from build123d import *

# Parameters (mm, degrees)
SKETCH1_W           = 250
SKETCH1_H           = 150
SKETCH1_R           = 6
BOSS_EXTRUDE1_DEPTH = 9.525
SKETCH2_W           = 9.525
SKETCH2_H           = 150
BOSS_EXTRUDE2_DEPTH = 200
SKETCH3_W           = 9.525
SKETCH3_H           = 150
BOSS_EXTRUDE3_DEPTH = 150


with BuildPart() as part:
    # Sketch1 → Boss-Extrude1 (new body)
    with BuildSketch(Plane.XY):
        with Locations((125, -75)):
            Rectangle(SKETCH1_W, SKETCH1_H)
        with Locations(Location((53.75, -40.75, 0), (0, 0, 180))):
            Circle(SKETCH1_R, mode=Mode.SUBTRACT)
        with Locations(Location((196.25, -40.75, 0), (0, 0, 180))):
            Circle(SKETCH1_R, mode=Mode.SUBTRACT)
        with Locations(Location((196.25, -109.25, 0), (0, 0, 180))):
            Circle(SKETCH1_R, mode=Mode.SUBTRACT)
        with Locations(Location((53.75, -109.25, 0), (0, 0, 180))):
            Circle(SKETCH1_R, mode=Mode.SUBTRACT)
    extrude(amount=BOSS_EXTRUDE1_DEPTH)

    # Sketch2 → Boss-Extrude2 (add)
    with BuildSketch(Plane.ZY):
        with Locations((4.7625, -75)):
            Rectangle(SKETCH2_W, SKETCH2_H)
    extrude(amount=BOSS_EXTRUDE2_DEPTH)

    # Sketch3 → Boss-Extrude3 (add)
    with BuildSketch(Plane(origin=(250, 0, 0), x_dir=(0, 0, -1), z_dir=(1, 0, 0))):
        with Locations((-4.7625, -75)):
            Rectangle(SKETCH3_W, SKETCH3_H)
    extrude(amount=BOSS_EXTRUDE3_DEPTH)


solid = part.part
Source: CAD feature listing. Evaluate the final solid. Frame: model axes, mm. Round coordinates to 2 decimals unless told otherwise and drop trailing zeros. Loops run counter-clockwise (first coordinate to the right, second up) from the corner with the lowest first, then second, coordinate; pieces in that order, holes last. Notation, with made-up numbers: (82.5, 15.25) - (139.5, 15.25) arc R21 ccw to (139.5, 52.25) - close; hole circle Ø5 at (-33, -8.5). An arc over 180 degrees is marked (long way). Write item = value, one per line. Start each with the question number.
Item 1: Section query A-A on y = -40.75. Output: boundary loops of the cut face in (x, z) (3 decimals), plus the area to 3 significant figures.
Item 2: Section query B-B on x = 53.75. Output: boundary loops of the cut face in (y, z) (3 decimals).
Item 3: Material intervals for line 1 (Y direction, x = 53.75, z = 4.75); line 2 (X direction, y = -40.75, z = 2.25); line 3 (X direction, y = -42.5, z = 4.5), sorted ascending.
Item 4: Mould query, pull axis X, two halves, no side actions, for faces 1 (the face through (96, 0, 5)), 2 (the face through (200.67, -113.31, 4.7)), 3 (the face through (-200, -74, 5)), 4 (the face through (54.53, -115.2, 4.7)). Classes: released by +X, released by -X, zero draft, split by the parting line, or undercut.
Results list:
q1.outline = (-200, 0) - (47.75, 0) - (47.75, 9.525) - (-200, 9.525) - close; (59.75, 0) - (190.25, 0) - (190.25, 9.525) - (59.75, 9.525) - close; (202.25, 0) - (400, 0) - (400, 9.525) - (202.25, 9.525) - close
q1.area = 5,490 mm²
q2.outline = (-150, 0) - (-115.25, 0) - (-115.25, 9.525) - (-150, 9.525) - close; (-103.25, 0) - (-46.75, 0) - (-46.75, 9.525) - (-103.25, 9.525) - close; (-34.75, 0) - (0, 0) - (0, 9.525) - (-34.75, 9.525) - close
q3.line_1 = -150 to -115.25, -103.25 to -46.75, -34.75 to 0
q3.line_2 = -200 to 47.75, 59.75 to 190.25, 202.25 to 400
q3.line_3 = -200 to 48.01, 59.49 to 190.51, 201.99 to 400
q4.face_1 = zero draft
q4.face_2 = undercut
q4.face_3 = released by -X
q4.face_4 = undercut
